Source: CAD feature listing. Evaluate the final solid. Frame: model axes, mm. A direction names the side the tool comes from. Give positions to 0.01 mm unless a question says otherwise; leave off trailing zeros. Write each loop counter-clockwise with the first axis right and the second up, starting at its lowest first coordinate (ties: lowest second). Pieces come first, ordered by that corner, then holes. Notation, with made-up numbers: M -9.5,83 L 41.5,83 A18 ccw 41.5,89 Z; hole C -21.5,83.5 d8. An arc over 180 degrees is marked long. Return JSON: item names as keys, results as strings.
```python
from build123d import *

# Parameters (mm, degrees)
SKETCH1_W                 = 210
SKETCH1_H                 = 12
BOSS_EXTRUDE1_DEPTH       = 116
SKETCH2_R                 = 10
CUT_EXTRUDE1_DEPTH        = 13
F_5_0MM_DOWEL_HOLE1_D     = 5
F_5_0MM_DOWEL_HOLE1_DEPTH = 25
F_5_0MM_DOWEL_HOLE1_TIP   = 1.502151548
F_5_0MM_DOWEL_HOLE2_D     = 5
F_5_0MM_DOWEL_HOLE2_DEPTH = 25
F_5_0MM_DOWEL_HOLE2_TIP   = 1.502151548
SKETCH7_R                 = 10
CUT_EXTRUDE2_DEPTH        = 13.0000001
SKETCH8_R                 = 15
CUT_EXTRUDE3_DEPTH        = 8
F_5_0MM_DOWEL_HOLE3_D     = 5
F_5_0MM_DOWEL_HOLE3_DEPTH = 12
F_5_0MM_DOWEL_HOLE3_TIP   = 1.502151548
F_5_0MM_DOWEL_HOLE4_D     = 5
F_5_0MM_DOWEL_HOLE4_DEPTH = 25
F_5_0MM_DOWEL_HOLE4_TIP   = 1.502151548


with BuildPart() as part:
    # Sketch1 → Boss-Extrude1 (new body)
    with BuildSketch(Plane(origin=(0, 0, 0), x_dir=(1, 0, 0), z_dir=(0, 1, 0))):
        with Locations((105, 6)):
            Rectangle(SKETCH1_W, SKETCH1_H)
    extrude(amount=BOSS_EXTRUDE1_DEPTH)

    # Sketch2 → Cut-Extrude1 (cut, through all)
    with BuildSketch(Plane.XY):
        with Locations((23, 55)):
            Circle(SKETCH2_R)
        with Locations((187, 55)):
            Circle(SKETCH2_R)
    extrude(amount=-CUT_EXTRUDE1_DEPTH, mode=Mode.SUBTRACT)

    # Ø5.0mm Dowel Hole1
    with Locations(Plane.ZY):
        with Locations((-6, 55)):
            Hole(F_5_0MM_DOWEL_HOLE1_D / 2, depth=F_5_0MM_DOWEL_HOLE1_DEPTH)
            with Locations((0, 0, -(F_5_0MM_DOWEL_HOLE1_DEPTH + F_5_0MM_DOWEL_HOLE1_TIP / 2))):  # 118° drill point
                Cone(0, F_5_0MM_DOWEL_HOLE1_D / 2, F_5_0MM_DOWEL_HOLE1_TIP, mode=Mode.SUBTRACT)

    # Ø5.0mm Dowel Hole2
    with Locations(Plane(origin=(210, 0, 0), x_dir=(0, 0, -1), z_dir=(1, 0, 0))):
        with Locations((6, 55)):
            Hole(F_5_0MM_DOWEL_HOLE2_D / 2, depth=F_5_0MM_DOWEL_HOLE2_DEPTH)
            with Locations((0, 0, -(F_5_0MM_DOWEL_HOLE2_DEPTH + F_5_0MM_DOWEL_HOLE2_TIP / 2))):  # 118° drill point
                Cone(0, F_5_0MM_DOWEL_HOLE2_D / 2, F_5_0MM_DOWEL_HOLE2_TIP, mode=Mode.SUBTRACT)

    # Sketch7 → Cut-Extrude2 (cut, through all)
    with BuildSketch(Plane.XY):
        with Locations((105, 55)):
            Circle(SKETCH7_R)
    extrude(amount=-CUT_EXTRUDE2_DEPTH, mode=Mode.SUBTRACT)

    # Sketch8 → Cut-Extrude3 (cut)
    with BuildSketch(Plane.XY):
        with Locations((105, 55)):
            Circle(SKETCH8_R)
    extrude(amount=-CUT_EXTRUDE3_DEPTH, mode=Mode.SUBTRACT)

    # Ø5.0mm Dowel Hole3
    with Locations(Plane(origin=(0, 0, 0), x_dir=(-1, 0, 0), z_dir=(0, -1, 0))):
        with Locations((-25, 6), (-105, 6), (-185, 6)):
            Hole(F_5_0MM_DOWEL_HOLE3_D / 2, depth=F_5_0MM_DOWEL_HOLE3_DEPTH)
            with Locations((0, 0, -(F_5_0MM_DOWEL_HOLE3_DEPTH + F_5_0MM_DOWEL_HOLE3_TIP / 2))):  # 118° drill point
                Cone(0, F_5_0MM_DOWEL_HOLE3_D / 2, F_5_0MM_DOWEL_HOLE3_TIP, mode=Mode.SUBTRACT)

    # Ø5.0mm Dowel Hole4
    with Locations(Plane(origin=(0, 0, -12), x_dir=(-1, 0, 0), z_dir=(0, 0, -1))):
        with Locations((-148, 55), (-62, 55)):
            Hole(F_5_0MM_DOWEL_HOLE4_D / 2, depth=F_5_0MM_DOWEL_HOLE4_DEPTH)
            with Locations((0, 0, -(F_5_0MM_DOWEL_HOLE4_DEPTH + F_5_0MM_DOWEL_HOLE4_TIP / 2))):  # 118° drill point
                Cone(0, F_5_0MM_DOWEL_HOLE4_D / 2, F_5_0MM_DOWEL_HOLE4_TIP, mode=Mode.SUBTRACT)


solid = part.part
```
1) Line query: line 1 (Y direction, x = 187, z = -8.75); line 2 (Z direction, x = 25, y = 3.25); line 3 (Y direction, x = 8, z = -6). Output: solid intervals per line, ascending. Write a range as [from, to].
Numbers:
{"line 1": "y = [0, 45], [65, 116]", "line 2": "z = [-12, -8.5], [-3.5, 0]", "line 3": "y = [0, 52.5], [57.5, 116]"}
2) Cut plane A-A, the plane x = 148. Return the cut outline in (y, z).
Numbers:
{"outline": "M 0,-12 L 52.5,-12 L 52.5,0 L 0,0 Z; M 57.5,-12 L 116,-12 L 116,0 L 57.5,0 Z"}
3) Set-up query: faces 1 (the face through (203.248, 55.751, -3.615)), 2 (the face through (107.385, 6.084, -6.751)), 3 (the face through (6.752, 55.751, -8.385)), 4 (the face through (119.307, 59.506, -3.944)). Return all of +Z, -Z, +X, -X, +Y, -Y with unobstructed straight access to the full face (end or side cutting, diameter ignored); none if empty.
Numbers:
{"face 1": "+X", "face 2": "-Y", "face 3": "-X", "face 4": "+Z"}
4) Cut plane B-B, the plane y = 55. Give the number of separate pieces and of enclosed holes in the cut face, then the cut area to 3 significant figures.
Numbers:
{"separate pieces": "8", "enclosed holes": "0", "area": "1,470 mm²"}
5) Contact query for flat-ended pins moving along their axis: pin 1 Ø6 at (y, z) = (83, -6.5) entering from -X; pin 2 Ø3 at (x, z) = (105, -6) entering from -Y; pin 3 Ø4 at (x, y) = (62, 55) entering from +Z; pin 4 Ø9 at (x, y) = (99.5, 62.5) entering from +Z. Output: stop coordinate, or through.
Numbers:
{"pin 1": "stops at x = 0", "pin 2": "stops at y = 12.6", "pin 3": "passes through", "pin 4": "stops at z = -8"}
6) Draft query along X for faces 5 (the face through (32.237, 51.17, -5.916)), 6 (the face through (210, 57, -3)), 7 (the face through (104, 0, -9)). Return one class per face: released by +X, released by -X, zero draft, split by the parting line, or undercut.
Numbers:
{"face 5": "undercut", "face 6": "released by +X", "face 7": "zero draft"}
